Build history of the part. All positions in model axes, mm. A direction names the side the tool comes from. Coordinates: 2 decimals unless noted, no trailing zeros. Loops run counter-clockwise (first coordinate to the right, second up) from the corner with the lowest first, then second, coordinate; pieces in that order, holes last. Notation, with made-up numbers: (-10.5, 5) - (41.5, 5) arc R17 cw to (41.5, 17) - close; hole circle Ø7 at (62, -18.75). An arc over 180 degrees is marked (long way). One line per item, written item: value.
```python
from build123d import *

# Parameters (mm, degrees)
EXTRUDE_958_DEPTH      = 8
SKETCH_5_R             = 1.25
CUT_EXTRUDE_1488_DEPTH = 13
SKETCH_6_R             = 1.25
CUT_EXTRUDE_1665_DEPTH = 10
FILLET_2_R             = 5


with BuildPart() as part:
    # Эскиз1 → Extrude 958 (new body)
    with BuildSketch(Plane.XY):
        Polygon((-20, 22), (-20, -22), (-10, -22), (20, 12), (20, 22), align=None)
        with BuildLine():
            Line((-12, 19), (-12, -14.442810634))
            ThreePointArc((-12, -14.442810634), (-10.707336051, -16.313552656), (-8.500324289, -15.766053908))
            Line((-8.500324289, -15.766053908), (12, 7.467646953))
            Line((12, 7.467646953), (12, 19))
            Line((12, 19), (-12, 19))
        make_face(mode=Mode.SUBTRACT)
    extrude(amount=EXTRUDE_958_DEPTH)

    # Эскиз5 → Cut-Extrude 1488 (cut)
    with BuildSketch(Plane.XZ.offset(22)):
        with Locations((-16, 4)):
            Circle(SKETCH_5_R)
    cut_extrude_1488 = extrude(amount=-CUT_EXTRUDE_1488_DEPTH, mode=Mode.SUBTRACT)

    # Эскиз6 → Cut-Extrude 1665 (cut)
    with BuildSketch(Plane(origin=(0, 22, 0), x_dir=(1, 0, 0), z_dir=(0, 1, 0))):
        with Locations(Location((16, -4, 0), (0, 0, 270))):
            Circle(SKETCH_6_R)
    extrude(amount=-CUT_EXTRUDE_1665_DEPTH, mode=Mode.SUBTRACT)

    # Скругление2
    fillet_2_edges = [part.edges().sort_by_distance(p)[0] for p in [
        (20, 12, 4),
    ]]
    fillet(fillet_2_edges, radius=FILLET_2_R)

    # Зеркальное отражение1: Cut-Extrude 1488 across plane
    add(cut_extrude_1488.mirror(Plane.ZX), mode=Mode.SUBTRACT)


solid = part.part
```
Item 1: Cut at B-B, the plane z = 4. Write the cut outline in (x, y), then the cut area to 3 significant figures.
Check result:
outline: (-20, -22) - (-17.25, -22) - (-17.25, -9) - (-14.75, -9) - (-14.75, -22) - (-10, -22) - (18.75, 10.58) arc R5 ccw to (20, 13.89) - (20, 22) - (17.25, 22) - (17.25, 12) - (14.75, 12) - (14.75, 22) - (-14.75, 22) - (-14.75, 9) - (-17.25, 9) - (-17.25, 22) - (-20, 22) - close; hole (-12, -14.44) arc R2 ccw to (-8.5, -15.77) - (12, 7.47) - (12, 19) - (-12, 19) - close
area: 562 mm^2
Item 2: Cut at C-C, the plane y = -6. Write the cut outline in (x, z), then the cut area to 3 significant figures.
Check result:
outline: (-20, 0) - (-12, 0) - (-12, 8) - (-20, 8) - close; (0.12, 0) - (4.12, 0) - (4.12, 8) - (0.12, 8) - close
area: 96.0 mm^2
Item 3: Pull direction Z, two halves, no side cores. Call faces 6 (the face through (-14, 5, 8)), 7 (the face through (-10.74, -16.3, 3.94)), 8 (the face through (17.054, 17.07, 4.672)): released by +Z, released by -Z, zero draft, split by the parting line, or undercut.
Check result:
face 6: released by +Z
face 7: zero draft
face 8: undercut
Item 4: Drop flat-ended pins along their axis: P1, Ø1.5, axis at x = 3.5, z = 3.5, coming from the -Y side; P2, Ø3, axis at x = -16, z = 4, coming from the -Y side; P3, Ø3, axis at y = 6.5, z = 2.5, coming from the +X side; P4, Ø2, axis at x = -16, z = 4, coming from the +Y side. Give the stop position or say it passes through.
Check result:
P1: stops at y = -7.55
P2: stops at y = -22
P3: stops at x = 16.47
P4: stops at y = 9
Item 5: Cut at A-A, the plane y = 15. Write the cut outline in (x, z), then the cut area to 3 significant figures.
Check result:
outline: (-20, 0) - (-12, 0) - (-12, 8) - (-20, 8) - close; (12, 0) - (20, 0) - (20, 8) - (12, 8) - close; hole circle Ø2.5 at (-16, 4); hole circle Ø2.5 at (16, 4)
area: 118 mm^2
Item 6: Cut at D-D, the plane x = -1. Write the cut outline in (y, z), then the cut area to 3 significant figures.
Check result:
outline: (-11.8, 0) - (-7.27, 0) - (-7.27, 8) - (-11.8, 8) - close; (19, 0) - (22, 0) - (22, 8) - (19, 8) - close
area: 60.3 mm^2
Item 7: Probe probe 1 along X at (y, z) = (16, 7.5); probe 2 along Z at (x, y) = (-16, -14); probe 3 along X at (y, z) = (17.5, 5). List the from-to ranges inside material, lowest first. Write a range as from..to.
Check result:
probe 1: x = -20..-12, 12..20
probe 2: z = 0..2.75, 5.25..8
probe 3: x = -20..-16.75, -15.25..-12, 12..15.25, 16.75..20
Item 8: Tool access for faces 1 (the face through (0, 19, 4)), 2 (the face through (-16, -9, 4)), 3 (the face through (4.17, -5.94, 3.94)), 4 (the face through (0, 22, 4)), 5 (the face through (-16, 9, 4)): list every direction of +Z, -Z, +X, -X, +Y, -Y with a clear straight run to the whole face (end or side of a thin tool).
Check result:
face 1: +Z, -Z
face 2: -Y
face 3: +Z, -Z, +X, -Y
face 4: +Z, -Z, +X, -X, +Y
face 5: +Y
